Read the model definition and answer for the solid it produces. Units are mm, in the model's axes. A direction names the side the tool comes from. Round coordinates to 2 decimals unless told otherwise and drop trailing zeros. Order: outer loops, then holes, each group sorted by start corner. A loop starts at its lowest first (then second) coordinate and runs counter-clockwise, first axis right, second up. Notation, with made-up numbers: (61.5, 66) - (118.5, 66) arc R23 cw to (118.5, 90) - close; hole circle Ø1 at (-24.75, -8.75). An arc over 180 degrees is marked (long way). Put each result on its own line as item: value. Start each with the question number.
Q1. Section B-B on x = 0 is taken. Give the vertices of the cut face in (y, z).
Q2. Section A-A on z = 0 is taken. Give the vertices of the cut face in (x, y).
Q3. Which of the six approach directions +Z, -Z, +X, -X, +Y, -Y give full straight-line access (tool end or side, diameter ignored) to faces 4 (the face through (0.33, 34.93, -7.493)), 5 (the face through (5.024, 19.86, -23.553)), 6 (the face through (22.225, 19.86, 3.506)), 7 (the face through (-22.01, 19.86, -9.78))?
Q4. For a pull along Z with two mould halves and no side action, classify faces 1 (the face through (-5.024, 19.86, -23.553)), 2 (the face through (24.241, 20.14, 7.913)), 3 (the face through (-23.553, 19.86, -5.024)) as pulls with the +Z half, pulls with the -Z half, needs draft (parallel to the pull), parting line crosses it, or undercut.
Q5. Section C-C on y = 6 is taken. Give the vertices of the cut face in (x, z), then the cut area to 3 significant figures.
Q6. Section D-D on z = -14.5 is taken. Give the vertices of the cut face in (x, y).
Q7. Find the intervals of material crossed by line 1 along Y through (x, z) = (15.5, 14); line 2 along Z through (x, y) = (-21.5, 21.5); line 3 along X through (y, z) = (20, -21), in increasing order. Write a range as from..to.
Q8. Each of these flat-tipped pins is pushed along its axis until it touches: pin 1 Ø2 at (x, y) = (1.5, 5) entering from -Z; pin 2 Ø3.5 at (x, y) = (-24, 19.5) entering from +Z; pin 3 Ø8 at (x, z) = (-14.5, 19.5) entering from +Y; pin 4 Ø12 at (x, y) = (1.5, 8) entering from +Z. Where does it stop, or does it pass through?
from build123d import *

# Parameters (mm, degrees)
ESQUISSE1_R                  = 7.5
BOSS_EXTRU_1_DEPTH           = 40
ESQUISSE2_R                  = 22.5
BOSS_EXTRU_2_DEPTH           = 20
ESQUISSE3_W                  = 5
ESQUISSE3_H                  = 20
BOSS_EXTRU_3_DEPTH           = 3
R_P_TITION_CIRCULAIRE4_COUNT = 20


with BuildPart() as part:
    # Esquisse1 → Boss.-Extru.1 (new body)
    with BuildSketch(Plane(origin=(0, 0, 0), x_dir=(1, 0, 0), z_dir=(0, 1, 0))):
        with Locations(Location((0, 0, 0), (0, 0, 270))):
            Circle(ESQUISSE1_R)
    extrude(amount=BOSS_EXTRU_1_DEPTH)

    # Esquisse2 → Boss.-Extru.2 (add)
    with BuildSketch(Plane(origin=(0, 10, 0), x_dir=(-1, 0, 0), z_dir=(0, -1, 0))):
        with Locations(Location((0, 0, 0), (0, 0, 90))):
            Circle(ESQUISSE2_R)
    extrude(amount=-BOSS_EXTRU_2_DEPTH)

    # Esquisse3 → Boss.-Extru.3 (add, symmetric)
    with BuildSketch(Plane.XY.offset(22.5)):
        with Locations((0, 20)):
            Rectangle(ESQUISSE3_W, ESQUISSE3_H)
    boss_extru_3 = extrude(amount=BOSS_EXTRU_3_DEPTH, both=True)

    # Répétition circulaire4: Boss.-Extru.3 ×20 about axis
    r_p_tition_circulaire4_axis = Axis((0, 0, 0), (0, 1, 0))
    for i in range(1, R_P_TITION_CIRCULAIRE4_COUNT):
        add(boss_extru_3.rotate(r_p_tition_circulaire4_axis, i * 360 / R_P_TITION_CIRCULAIRE4_COUNT))


solid = part.part
Findings:
1. outline: (0, -7.5) - (10, -7.5) - (10, -25.5) - (30, -25.5) - (30, -7.5) - (40, -7.5) - (40, 7.5) - (30, 7.5) - (30, 25.5) - (10, 25.5) - (10, 7.5) - (0, 7.5) - close
2. outline: (-25.5, 10) - (-7.5, 10) - (-7.5, 0) - (7.5, 0) - (7.5, 10) - (25.5, 10) - (25.5, 30) - (7.5, 30) - (7.5, 40) - (-7.5, 40) - (-7.5, 30) - (-25.5, 30) - close
3. face 4: +Y
3. face 5: -Z, +Y, -Y
3. face 6: +X, +Y, -Y
3. face 7: +Y, -Y
4. face 1: pulls with the -Z half
4. face 2: pulls with the +Z half
4. face 3: undercut
5. outline: circle Ø15 at (0, 0)
5. area: 177 mm2
6. outline: (-20.98, 10) - (20.98, 10) - (20.98, 30) - (-20.98, 30) - close
7. line 1: 10..30
7. line 2: -13.79..-12.53, -9.61..9.61, 12.53..13.79
7. line 3: -14.48..-12.17, -9.45..9.45, 12.17..14.48
8. pin 1: z = -7.48
8. pin 2: z = 10.26
8. pin 3: y = 30
8. pin 4: z = 25.5
